Read the model definition and answer for the solid it produces. Units are mm, in the model's axes. Face numbers are marked on the shaded views. A direction names the side the tool comes from. Give positions to 0.01 mm unless a question says otherwise; leave off trailing zeros. Order: outer loops, then holes, each group sorted by start corner. A loop starts at its lowest first (then second) coordinate and runs counter-clockwise, first axis right, second up. Notation, with made-up numbers: (-31.5, 72) - (16.5, 72) arc R30 cw to (16.5, 107) - close; hole circle Ø9 at (-32.75, 19.5). An arc over 180 degrees is marked (long way). Write each question's results on one line, items separated by ' | '.
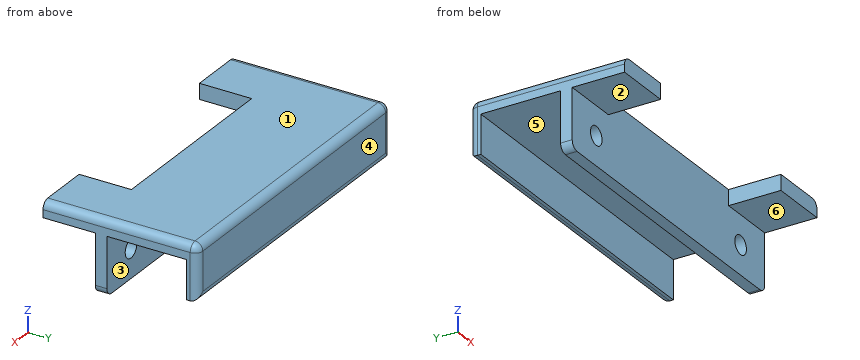
from build123d import *

# Parameters (mm, degrees)
SKETCH_1_R              = 1.7
SKETCH_1_R_2            = 11.5
EXTRUDE_1_DEPTH         = 4
SKETCH_1_4_W            = 80
SKETCH_1_4_H            = 3
EXTRUDE_2_DEPTH         = 10
EXTRUDE_3_DEPTH         = 10
RIB_2_REACH             = 110.093
SKETCH_4_WALL_W         = 240.545785644
SKETCH_4_WALL_H         = 5
SKETCH_5_W              = 2
SKETCH_5_H              = 0.1
SKETCH_5_W_2            = 4.2
SKETCH_5_H_2            = 2
CUT_EXTRUDE_2_DEPTH     = 10
CHAMFER_1_SIZE          = 0.25
SKETCH_6_W              = 91
SKETCH_6_H              = 17
EXTRUDE_4_DEPTH         = 4
SKETCH_7_W              = 80
SKETCH_7_H              = 3.5
EXTRUDE_5_DEPTH         = 15
SKETCH_8_W              = 50
SKETCH_8_H              = 13.5
CUT_EXTRUDE_3_DEPTH     = 102.533245787
CUT_EXTRUDE_4_DEPTH     = 15
CUT_EXTRUDE_5_REACH     = 113.513
SKETCH_10_R             = 2.4
FILLET_1_R              = 10
SKETCH_11_W             = 92.157342817
SKETCH_11_H             = 59.862511732
CUT_EXTRUDE_6_DEPTH     = 103.200782776
CUT_EXTRUDE_START       = -15
CUT_EXTRUDE_7_OUTLINE_W = 80
CUT_EXTRUDE_7_OUTLINE_H = 0.5
CUT_EXTRUDE_7_DEPTH     = 15
FILLET_2_R              = 2


# Read off the part's stored shape, not the designer's step: 切除-拉伸7
with BuildPart() as part:
    # 草图1 → 凸台-拉伸1 (new body)
    with BuildSketch(Plane.XY):
        with BuildLine():
            Line((-70, 13), (-70, -10))
            Line((-70, -10), (21, -10))
            Line((21, -10), (21, 44.755002002))
            ThreePointArc((21, 44.755002002), (20.506939094, 46.920065511), (19.125, 48.658125751))
            ThreePointArc((19.125, 48.658125751), (18, 51), (19.125, 53.341874249))
            ThreePointArc((19.125, 53.341874249), (20.506939094, 55.079934489), (21, 57.244997998))
            Line((21, 57.244997998), (21, 67))
            ThreePointArc((21, 67), (19.535533906, 70.535533906), (16, 72))
            Line((16, 72), (6.244997998, 72))
            ThreePointArc((6.244997998, 72), (4.079934489, 71.506939094), (2.341874249, 70.125))
            ThreePointArc((2.341874249, 70.125), (0, 69), (-2.341874249, 70.125))
            ThreePointArc((-2.341874249, 70.125), (-4.079934489, 71.506939094), (-6.244997998, 72))
            Line((-6.244997998, 72), (-16, 72))
            ThreePointArc((-16, 72), (-19.535533906, 70.535533906), (-21, 67))
            Line((-21, 67), (-21, 57.244997998))
            ThreePointArc((-21, 57.244997998), (-20.506939094, 55.079934489), (-19.125, 53.341874249))
            ThreePointArc((-19.125, 53.341874249), (-18, 51), (-19.125, 48.658125751))
            ThreePointArc((-19.125, 48.658125751), (-20.506939094, 46.920065511), (-21, 44.755002002))
            Line((-21, 44.755002002), (-21, 13))
            Line((-21, 13), (-70, 13))
        make_face()
        with Locations((-15.5, 35.5)):
            Circle(SKETCH_1_R, mode=Mode.SUBTRACT)
        with Locations((-15.5, 66.5)):
            Circle(SKETCH_1_R, mode=Mode.SUBTRACT)
        with Locations((15.5, 35.5)):
            Circle(SKETCH_1_R, mode=Mode.SUBTRACT)
        with Locations((0, 51)):
            Circle(SKETCH_1_R_2, mode=Mode.SUBTRACT)
        with Locations((15.5, 66.5)):
            Circle(SKETCH_1_R, mode=Mode.SUBTRACT)
    extrude(amount=EXTRUDE_1_DEPTH)

    # 草图1<4> → 凸台-拉伸2 (add)
    with BuildSketch(Plane.XY):
        with Locations((-30, 11.5)):
            Rectangle(SKETCH_1_4_W, SKETCH_1_4_H)
    extrude(amount=-EXTRUDE_2_DEPTH)

    # 草图1<5> → 凸台-拉伸3 (add)
    with BuildSketch(Plane.XY):
        Polygon((3.05, 8), (3.05, 10), (-3.05, 10), (-3.05, 8), (-5.05, 8), (-5.05, 6.5), (-4.55, 6), (4.55, 6), (5.05, 6.5), (5.05, 8), align=None)
        Polygon((-16.95, 10), (-23.05, 10), (-23.05, 8), (-25.05, 8), (-25.05, 6.5), (-24.55, 6), (-15.45, 6), (-14.95, 6.5), (-14.95, 8), (-16.95, 8), align=None)
        Polygon((-36.95, 10), (-43.05, 10), (-43.05, 8), (-45.05, 8), (-45.05, 6.5), (-44.55, 6), (-35.45, 6), (-34.95, 6.5), (-34.95, 8), (-36.95, 8), align=None)
        Polygon((-26, 4.55), (-26, -4.55), (-26.5, -5.05), (-28, -5.05), (-28, -3.05), (-32, -3.05), (-32, -5.05), (-33.5, -5.05), (-34, -4.55), (-34, 4.55), (-33.5, 5.05), (-32, 5.05), (-32, 3.05), (-28, 3.05), (-28, 5.05), (-26.5, 5.05), align=None)
        Polygon((-23.05, -8), (-23.05, -10), (-16.95, -10), (-16.95, -8), (-14.95, -8), (-14.95, -6.5), (-15.45, -6), (-24.55, -6), (-25.05, -6.5), (-25.05, -8), align=None)
        Polygon((-43.05, -8), (-43.05, -10), (-36.95, -10), (-36.95, -8), (-34.95, -8), (-34.95, -6.5), (-35.45, -6), (-44.55, -6), (-45.05, -6.5), (-45.05, -8), align=None)
    extrude(amount=-EXTRUDE_3_DEPTH)

    # 草图4 wall → 筋2 (add, up to next)
    with BuildSketch(Plane(origin=(10, 23, -5), x_dir=(0, 0.894427191, 0.4472135955), z_dir=(0, -0.4472135955, 0.894427191)), mode=Mode.PRIVATE) as rib_2_sk1:
        with Locations((0, 2.5)):
            Rectangle(SKETCH_4_WALL_W, SKETCH_4_WALL_H)
    rib_2_tool1 = extrude(rib_2_sk1.sketch, amount=RIB_2_REACH, mode=Mode.PRIVATE) - part.part
    rib_2 = rib_2_tool1.solids().sort_by_distance((10, 23, -5))[0]
    add(rib_2)

    # 镜向1: 筋2 across plane
    add(rib_2.mirror(Plane(origin=(0, 0, 0), x_dir=(0, 0, 1), z_dir=(1, 0, 0))))

    # 草图5 → 切除-拉伸2 (cut)
    with BuildSketch(Plane(origin=(0, 0, -10), x_dir=(-1, 0, 0), z_dir=(0, 0, -1))):
        with Locations((15.95, 7.95)):
            Rectangle(SKETCH_5_W, SKETCH_5_H)
        with Locations((24.05, 7.95)):
            Rectangle(SKETCH_5_W, SKETCH_5_H)
        with Locations((35.95, 7.95)):
            Rectangle(SKETCH_5_W, SKETCH_5_H)
        with Locations((44.05, 7.95)):
            Rectangle(SKETCH_5_W, SKETCH_5_H)
        with Locations((30, 4.05)):
            Rectangle(SKETCH_5_W_2, SKETCH_5_H_2)
        with Locations((30, -4.05)):
            Rectangle(SKETCH_5_W_2, SKETCH_5_H_2)
        with Locations((44.05, -7.95)):
            Rectangle(SKETCH_5_W, SKETCH_5_H)
        with Locations((35.95, -7.95)):
            Rectangle(SKETCH_5_W, SKETCH_5_H)
        with Locations((24.05, -7.95)):
            Rectangle(SKETCH_5_W, SKETCH_5_H)
        with Locations((15.95, -7.95)):
            Rectangle(SKETCH_5_W, SKETCH_5_H)
    extrude(amount=-CUT_EXTRUDE_2_DEPTH, mode=Mode.SUBTRACT)

    # 倒角1
    chamfer_1_edges = [part.edges().sort_by_distance(p)[0] for p in [
        (3.05, 8, -5),
        (5.05, 8, -5),
        (-5.05, 8, -5),
        (-3.05, 8, -5),
        (-16.95, 7.9, -5),
        (-14.95, 7.9, -5),
        (-23.05, 7.9, -5),
        (-25.05, 7.9, -5),
        (-36.95, 7.9, -5),
        (-34.95, 7.9, -5),
        (-43.05, 7.9, -5),
        (-45.05, 7.9, -5),
        (-27.9, 5.05, -5),
        (-32.1, 3.05, -5),
        (-32.1, 5.05, -5),
        (-27.9, 3.05, -5),
        (-32.1, -5.05, -5),
        (-32.1, -3.05, -5),
        (-27.9, -3.05, -5),
        (-27.9, -5.05, -5),
        (-43.05, -7.9, -5),
        (-45.05, -7.9, -5),
        (-36.95, -7.9, -5),
        (-34.95, -7.9, -5),
        (-23.05, -7.9, -5),
        (-25.05, -7.9, -5),
        (-16.95, -7.9, -5),
        (-14.95, -7.9, -5),
    ]]
    chamfer(chamfer_1_edges, length=CHAMFER_1_SIZE)

    # 草图6 → 凸台-拉伸4 (add)
    with BuildSketch(Plane.XY.offset(4)):
        with Locations((-24.5, -18.5)):
            Rectangle(SKETCH_6_W, SKETCH_6_H)
    extrude(amount=-EXTRUDE_4_DEPTH)

    # 草图7 → 凸台-拉伸5 (add)
    with BuildSketch(Plane(origin=(0, 0, 0), x_dir=(-1, 0, 0), z_dir=(0, 0, -1))):
        with Locations((30, -11.75)):
            Rectangle(SKETCH_7_W, SKETCH_7_H)
    extrude(amount=EXTRUDE_5_DEPTH)

    # 草图8 → 切除-拉伸3 (cut, through all)
    with BuildSketch(Plane(origin=(0, 0, 0), x_dir=(-1, 0, 0), z_dir=(0, 0, -1))):
        with Locations((30, -20.25)):
            Rectangle(SKETCH_8_W, SKETCH_8_H)
        with BuildLine():
            Line((-21, -27), (-10, -27))
            Line((-10, -27), (-10, 26))
            ThreePointArc((-10, 26), (-11.171572875, 28.828427125), (-14, 30))
            Line((-14, 30), (-16, 30))
            ThreePointArc((-16, 30), (-19.535533906, 31.464466094), (-21, 35))
            Line((-21, 35), (-21, 30))
            Line((-21, 30), (-21, -27))
        make_face()
    extrude(amount=-CUT_EXTRUDE_3_DEPTH, mode=Mode.SUBTRACT)

    # 草图9 → 切除-拉伸4 (cut)
    with BuildSketch(Plane(origin=(0, 0, -15), x_dir=(-1, 0, 0), z_dir=(0, 0, -1))):
        Polygon((50, -10), (25.452851286, -10), (11.122555598, -10), (11.122555598, 0.364824121), (25.452851286, 0.364824121), (25.452851286, 5.586221175), (50, 5.586221175), align=None)
    extrude(amount=-CUT_EXTRUDE_4_DEPTH, mode=Mode.SUBTRACT)

    # 草图10 → 切除-拉伸5 (cut, up to next)
    with BuildSketch(Plane.XZ.offset(13.5), mode=Mode.PRIVATE) as cut_extrude_5_sk1:
        with Locations(Location((0, -7.5, 0), (0, 0, 270))):
            Circle(SKETCH_10_R)
    cut_extrude_5_tool1 = extrude(cut_extrude_5_sk1.sketch, amount=-CUT_EXTRUDE_5_REACH, mode=Mode.PRIVATE) & part.part
    # 草图10 → 切除-拉伸5 (cut, up to next)
    with BuildSketch(Plane.XZ.offset(13.5), mode=Mode.PRIVATE) as cut_extrude_5_sk2:
        with Locations(Location((-60, -7.5, 0), (0, 0, 270))):
            Circle(SKETCH_10_R)
    cut_extrude_5_tool2 = extrude(cut_extrude_5_sk2.sketch, amount=-CUT_EXTRUDE_5_REACH, mode=Mode.PRIVATE) & part.part
    add(cut_extrude_5_tool1.solids().sort_by_distance((0, -13.5, -7.5))[0], mode=Mode.SUBTRACT)
    add(cut_extrude_5_tool2.solids().sort_by_distance((-60, -13.5, -7.5))[0], mode=Mode.SUBTRACT)

    # 圆角1
    fillet_1_edges = [part.edges().sort_by_distance(p)[0] for p in [
        (-21, 13, 2),
    ]]
    fillet(fillet_1_edges, radius=FILLET_1_R)

    # 草图11 → 切除-拉伸6 (cut, through all)
    with BuildSketch(Plane(origin=(0, 0, -15), x_dir=(-1, 0, 0), z_dir=(0, 0, -1))):
        with Locations((23.921328592, 42.931255866)):
            Rectangle(SKETCH_11_W, SKETCH_11_H)
    extrude(amount=-CUT_EXTRUDE_6_DEPTH, mode=Mode.SUBTRACT)

    # 切除-拉伸7 outline → 切除-拉伸7 (cut)
    with BuildSketch(Plane(origin=(0, 0, -15), x_dir=(-1, 0, 0), z_dir=(0, 0, -1)).offset(CUT_EXTRUDE_START)):
        with Locations((30, -10.25)):
            Rectangle(CUT_EXTRUDE_7_OUTLINE_W, CUT_EXTRUDE_7_OUTLINE_H)
        Polygon((-10, 10.1), (-10, 10), (-3.05, 10), (-3.05, 8.25), (-3.3, 8), (-4.8, 8), (-5.05, 7.75), (-5.05, 6.5), (-4.55, 6), (4.55, 6), (5.05, 6.5), (5.05, 7.75), (4.8, 8), (3.3, 8), (3.05, 8.25), (3.05, 10), (16.95, 10), (16.95, 8.15), (16.7, 7.9), (15.2, 7.9), (14.95, 7.65), (14.95, 6.5), (15.45, 6), (24.55, 6), (25.05, 6.5), (25.05, 7.65), (24.8, 7.9), (23.3, 7.9), (23.05, 8.15), (23.05, 10), (36.95, 10), (36.95, 8.15), (36.7, 7.9), (35.2, 7.9), (34.95, 7.65), (34.95, 6.5), (35.45, 6), (44.55, 6), (45.05, 6.5), (45.05, 7.65), (44.8, 7.9), (43.3, 7.9), (43.05, 8.15), (43.05, 10), (70, 10), (70, 10.1), align=None)
    extrude(amount=CUT_EXTRUDE_7_DEPTH, mode=Mode.SUBTRACT)

    # 圆角2
    fillet_2_edges = [part.edges().sort_by_distance(p)[0] for p in [
        (-70, 13, -3),
        (-70, -12, -15),
        (-30, 13, -10),
        (-70, -7, 4),
        (-30, 13, 4),
        (10, -7, 4),
        (10, 13, -3),
        (10, -12, -15),
    ]]
    fillet(fillet_2_edges, radius=FILLET_2_R)


solid = part.part
(1) Consider probe 1 along X at (y, z) = (-11.4, -7.5); probe 2 along Y at (x, z) = (-44, -6); probe 3 along X at (y, z) = (-19, 0.5). Determine where each line is inside the solid, lowest interval first. Write a range as [from, to].
Conclusion:
probe 1: [-70, -62.4], [-57.6, -2.4], [2.4, 10] | probe 2: [-13.5, -10.5], [10.1, 13] | probe 3: [-70, -55], [-5, 10]
(2) The mould has two halves that part along Y. Classify the marked faces 4, 5 and 6: pulls with the +Y half, pulls with the -Y half, needs draft (parallel to the pull), parting line crosses it, or undercut.
Conclusion:
face 4: pulls with the +Y half | face 5: undercut | face 6: needs draft
(3) Section D-D (x = -13.5) is taken. Give the vertices of the cut face in (y, z).
Conclusion:
outline: (-13.5, -15) - (-10.5, -15) - (-10.5, 0) - (10.1, 0) - (10.1, -10) - (11, -10) arc R2 ccw to (13, -8) - (13, 2) arc R2 ccw to (11, 4) - (-13.5, 4) - close
(4) Section A-A (x = -60) is taken. Give the vertices of the cut face in (y, z), plus the area to 3 significant figures.
Conclusion:
outline: (-27, 0) - (-13.5, 0) - (-13.5, -5.1) - (-10.5, -5.1) - (-10.5, 0) - (10.1, 0) - (10.1, -10) - (11, -10) arc R2 ccw to (13, -8) - (13, 2) arc R2 ccw to (11, 4) - (-27, 4) - close; (-13.5, -15) - (-10.5, -15) - (-10.5, -9.9) - (-13.5, -9.9) - close | area: 218 mm^2
(5) Section B-B (z = -1) is taken. Give the vertices of the cut face in (x, y), plus the area to 3 significant figures.
Conclusion:
outline: (-70, -13.5) - (10, -13.5) - (10, -10.5) - (-70, -10.5) - close; (-70, 10.1) - (10, 10.1) - (10, 11) arc R2 ccw to (8, 13) - (-68, 13) arc R2 ccw to (-70, 11) - close | area: 470 mm^2
(6) For the marked faces 1, 2 and 3, determine the directions among +Z, -Z, +X, -X, +Y, -Y from which every point of the face is accessible in a straight line to the end or side of a thin tool.
Conclusion:
face 1: +Z, +X, -X, +Y, -Y | face 2: -Z, +X, -X, -Y | face 3: -Z, +X, -X
(7) Section C-C (y = -17.5) is taken. Give the vertices of the cut face in (x, z), plus the area to 3 significant figures.
Conclusion:
outline: (-70, 0) - (-55, 0) - (-55, 4) - (-68, 4) arc R2 ccw to (-70, 2) - close; (-5, 0) - (10, 0) - (10, 2) arc R2 ccw to (8, 4) - (-5, 4) - close | area: 118 mm^2
(8) Each of these flat-tipped pins is pushed along its axis until it touches: pin 1 (6 mm diameter, centred on x = 0, z = -7.5, fed in from -Y); pin 2 (15 mm diameter, centred on x = -63, y = -23, fed in from -Z); pin 3 (1 mm diameter, centred on x = -43, y = 10.5, fed in from -Z). Where does it stop, or does it pass through?
Conclusion:
pin 1: y = -13.5 | pin 2: z = 0 | pin 3: z = -10
